Could you check a few things on this model? Use its own coordinates, in mm. A direction names the side the tool comes from. Coordinates: 2 decimals unless noted, no trailing zeros. Order: outer loops, then holes, each group sorted by start corner. A loop starts at its lowest first (then second) coordinate and runs counter-clockwise, first axis right, second up. Notation, with made-up numbers: (72.5, 76.5) -> (105.5, 76.5) arc R19 cw to (105.5, 82.5) -> close; hole circle Ø11 at (19.5, 85.5). An arc over 180 degrees is marked (long way). Use a Markdown table: item, result. Add a question column.
1) Thinking about a two-plate mould opening in Y: for faces 1 (the flat face through (-53.04, -42.24, -0.08)), 2 (the cylindrical face through (-19.527, 148.724, 0.112)), 3 (the flat face through (-91, -79, -23)), which applies, +Y half, -Y half, draft (parallel to the pull), parting line (faces both ways), or undercut?
2) If we section it at D-D (z = 61): Write out the boundary of the cut face in (x, y).
3) Which directions (+Z, -Z, +X, -X, +Y, -Y) give clear straight access to the entire face, cutting with the end or side of a thin tool? Please do faces 4 (the flat face through (56, 40, -6)), 5 (the flat face through (-56, -40, 6)), 6 (the flat face through (-61.43, -29.78, 0.08)).
4) Will these pins go through, and if not, where does the flat tip stop? pin 1 Ø1.5 at (y, z) = (19, -5.5) entering from +X; pin 2 Ø18 at (x, y) = (67.5, 43.5) entering from -Z; pin 3 Ø8 at (x, y) = (6.5, -46.5) entering from +Z.
5) If we section it at A-A (z = -1): Give the number of separate pieces and of enclosed holes in the cut face, plus the area to 3 significant figures.
6) If I drill on L1, parallel to Y at x = 0, z = 9; L2, parallel to X at y = 6, z = -14; L3, parallel to Y at x = 0, z = -11, over which ranges is the centre line in solid material (lowest first)? Write a range as [from, to].
```python
from build123d import *

# Parameters (mm, degrees)
SKETCH1_R           = 18
BOSS_EXTRUDE1_DEPTH = 37.5
SKETCH2_R           = 150
SKETCH2_R_2         = 120
BOSS_EXTRUDE2_DEPTH = 23
BOSS_EXTRUDE3_DEPTH = 6
CIRPATTERN15_COUNT  = 6
FILLET1_R           = 15
BOSS_EXTRUDE4_DEPTH = 42.5


with BuildPart() as part:
    # Sketch1 → Boss-Extrude1 (new, symmetric)
    with BuildSketch(Plane.XY):
        Circle(SKETCH1_R)
    extrude(amount=BOSS_EXTRUDE1_DEPTH, both=True)



with BuildPart() as body_2:
    # Sketch2 → Boss-Extrude2 (new, symmetric)
    with BuildSketch(Plane.XY):
        Circle(SKETCH2_R)
        Circle(SKETCH2_R_2, mode=Mode.SUBTRACT)
    extrude(amount=BOSS_EXTRUDE2_DEPTH, both=True)


with BuildPart() as part_1:
    add(part.part)

    add(body_2.part)  # Boss-Extrude3 merges body 2
    # Sketch3 → Boss-Extrude3 (add, symmetric)
    with BuildSketch(Plane.XY):
        with BuildLine():
            Line((-6.292975555, 119.834879975), (-1.969902622, 17.891883178))
            ThreePointArc((-1.969902622, 17.891883178), (-5.010440879, 17.288593991), (-7.902385067, 16.172578961))
            Line((-7.902385067, 16.172578961), (-12.278660753, 119.370157452))
            ThreePointArc((-12.278660753, 119.370157452), (-9.288724915, 119.639958164), (-6.292975555, 119.834879975))
        make_face()
        with BuildLine():
            Line((13.720864234, 119.212993774), (8.097322617, 16.075862852))
            ThreePointArc((8.097322617, 16.075862852), (5.2190816, 17.226757886), (2.18605888, 17.866760942))
            Line((2.18605888, 17.866760942), (7.741234625, 119.750045037))
            ThreePointArc((7.741234625, 119.750045037), (10.734408595, 119.51892098), (13.720864234, 119.212993774))
        make_face()
    boss_extrude3 = extrude(amount=BOSS_EXTRUDE3_DEPTH, both=True)

    # CirPattern15: Boss-Extrude3 ×6 about axis
    cirpattern15_axis = Axis((0, 0, 0), (0, 0, 1))
    for i in range(1, CIRPATTERN15_COUNT):
        add(boss_extrude3.rotate(cirpattern15_axis, i * 360 / CIRPATTERN15_COUNT))

    # Fillet1
    fillet1_edges = [part_1.edges().sort_by_distance(p)[0] for p in [
        (-150, 0, 23),
        (-150, 0, -23),
    ]]
    fillet(fillet1_edges, radius=FILLET1_R)

    # Sketch5 → Boss-Extrude4 (add)
    with BuildSketch(Plane.XY.offset(37.5)):
        with BuildLine():
            Line((-3.31662479, 5), (3.31662479, 5))
            ThreePointArc((3.31662479, 5), (6, 0), (3.31662479, -5))
            Line((3.31662479, -5), (-3.31662479, -5))
            ThreePointArc((-3.31662479, -5), (-6, 0), (-3.31662479, 5))
        make_face()
    boss_extrude4 = extrude(amount=BOSS_EXTRUDE4_DEPTH)

    # Mirror1: Boss-Extrude4 across plane
    add(boss_extrude4.mirror(Plane.XY))


solid = part_1.part
```
Answer sheet:
| question | item | result |
|---|---|---|
| 1 | face 1 | undercut |
| 1 | face 2 | parting line |
| 1 | face 3 | draft |
| 2 | outline | (-3.32, -5) -> (3.32, -5) arc R6 ccw to (3.32, 5) -> (-3.32, 5) arc R6 ccw to start |
| 3 | face 4 | -Z |
| 3 | face 5 | +Z |
| 3 | face 6 | +Z, -Z |
| 4 | pin 1 | x = 148.89 |
| 4 | pin 2 | z = -6 |
| 4 | pin 3 | z = 6 |
| 5 | separate pieces | 1 |
| 5 | enclosed holes | 12 |
| 5 | area | 33,800 mm2 |
| 6 | L1 | [-149.97, -120], [-18, 18], [120, 149.97] |
| 6 | L2 | [-148.63, -119.85], [-16.97, 16.97], [119.85, 148.63] |
| 6 | L3 | [-149.7, -120], [-18, 18], [120, 149.7] |
